Here's how the part is built. I have some questions about the finished solid (model axes, mm). A direction names the side the tool comes from. Round coordinates to 2 decimals unless told otherwise and drop trailing zeros. Write each loop counter-clockwise with the first axis right and the second up, starting at its lowest first coordinate (ties: lowest second). Pieces come first, ordered by that corner, then holes. Notation, with made-up numbers: (12.25, -34) - (36.25, -34) arc R23 cw to (36.25, -16) - close; hole circle Ø4 at (69.25, -3). An arc over 180 degrees is marked (long way). Return JSON: item names as keys, results as strings. Group by question number.
```python
from build123d import *

# Parameters (mm, degrees)
PAD_DEPTH       = 14
POCKET_DEPTH    = 13
SKETCH002_R     = 0.75
POCKET001_DEPTH = 5
SKETCH003_W     = 9
SKETCH003_H     = 54
PAD001_DEPTH    = 6
SKETCH004_R     = 1.6
POCKET002_DEPTH = 10
POCKET003_DEPTH = 4.5
CHAMFER001_SIZE = 1.5
CHAMFER003_SIZE = 0.25


with BuildPart() as part:
    # Sketch → Pad (new body)
    with BuildSketch(Plane.XY.offset(-6)):
        with BuildLine():
            ThreePointArc((-18.5, 103), (-23.449747, 100.949747), (-25.5, 96))
            Line((-25.5, 52), (-25.5, 96))
            ThreePointArc((-25.5, 52), (-23.449747, 47.050253), (-18.5, 45))
            Line((57.25, 45), (-18.5, 45))
            ThreePointArc((57.25, 45), (62.199747, 47.050253), (64.25, 52))
            Line((64.25, 96), (64.25, 52))
            ThreePointArc((64.25, 96), (62.199747, 100.949747), (57.25, 103))
            Line((-18.5, 103), (57.25, 103))
        make_face()
    extrude(amount=PAD_DEPTH)

    # Sketch001 → Pocket (cut)
    with BuildSketch(Plane.XY.offset(10)):
        with BuildLine():
            ThreePointArc((-18.5, 100.5), (-21.681981, 99.181981), (-23, 96))
            Line((-23, 52), (-23, 96))
            ThreePointArc((-23, 52), (-21.681981, 48.818019), (-18.5, 47.5))
            Line((57.25, 47.5), (-18.5, 47.5))
            ThreePointArc((57.25, 47.5), (60.431981, 48.818019), (61.75, 52))
            Line((61.75, 96), (61.75, 52))
            ThreePointArc((61.75, 96), (60.431981, 99.181981), (57.25, 100.5))
            Line((-18.5, 100.5), (57.25, 100.5))
        make_face()
    extrude(amount=-POCKET_DEPTH, mode=Mode.SUBTRACT)

    # Sketch002 → Pocket001 (cut)
    with BuildSketch(Plane(origin=(0, 104, 0), x_dir=(-1, 0, 0), z_dir=(0, 1, 0))):
        with Locations((-48.76875, 1.95)):
            Circle(SKETCH002_R)
        with Locations((-25.25, 1.95)):
            Circle(SKETCH002_R)
        with BuildLine():
            ThreePointArc((-40.17, 5.11), (-41.23066, 4.67066), (-41.67, 3.61))
            Line((-41.67, 3.05), (-41.67, 3.61))
            ThreePointArc((-41.67, 3.05), (-41.23066, 1.98934), (-40.17, 1.55))
            Line((-33.83, 1.55), (-40.17, 1.55))
            ThreePointArc((-33.83, 1.55), (-32.76934, 1.98934), (-32.33, 3.05))
            Line((-32.33, 3.61), (-32.33, 3.05))
            ThreePointArc((-32.33, 3.61), (-32.76934, 4.67066), (-33.83, 5.11))
            Line((-40.17, 5.11), (-33.83, 5.11))
        make_face()
        with BuildLine():
            ThreePointArc((-18.65, 14.05), (-19.286396, 13.786396), (-19.55, 13.15))
            Line((-19.55, 2.65), (-19.55, 13.15))
            ThreePointArc((-19.55, 2.65), (-19.286396, 2.013604), (-18.65, 1.75))
            Line((10.15, 1.75), (-18.65, 1.75))
            ThreePointArc((10.15, 1.75), (10.786396, 2.013604), (11.05, 2.65))
            Line((11.05, 13.15), (11.05, 2.65))
            ThreePointArc((11.05, 13.15), (10.786396, 13.786396), (10.15, 14.05))
            Line((-18.65, 14.05), (10.15, 14.05))
        make_face()
    extrude(amount=-POCKET001_DEPTH, mode=Mode.SUBTRACT)

    # Sketch003 → Pad001 (join)
    with BuildSketch(Plane.XY.offset(-6)):
        with Locations((-18.5, 74)):
            Rectangle(SKETCH003_W, SKETCH003_H)
        with Locations((57.25, 74)):
            Rectangle(SKETCH003_W, SKETCH003_H)
    extrude(amount=PAD001_DEPTH)

    # Sketch004 → Pocket002 (cut)
    with BuildSketch(Plane.XY):
        with Locations((-18.5, 96)):
            Circle(SKETCH004_R)
        with Locations((-18.5, 53)):
            Circle(SKETCH004_R)
        with Locations((57.25, 53)):
            Circle(SKETCH004_R)
        with Locations((57.25, 96)):
            Circle(SKETCH004_R)
    extrude(amount=-POCKET002_DEPTH, mode=Mode.SUBTRACT)

    # Sketch005 → Pocket003 (cut)
    with BuildSketch(Plane(origin=(0, 0, -6), x_dir=(-1, 0, 0), z_dir=(0, 0, -1))):
        Polygon((21.25, 94.412287), (21.25, 97.587713), (18.5, 99.175426), (15.75, 97.587713), (15.75, 94.412287), (18.5, 92.824574), align=None)
        Polygon((21.25, 51.412287), (21.25, 54.587713), (18.5, 56.175426), (15.75, 54.587713), (15.75, 51.412287), (18.5, 49.824574), align=None)
        Polygon((-54.5, 54.587713), (-57.25, 56.175426), (-60, 54.587713), (-60, 51.412287), (-57.25, 49.824574), (-54.5, 51.412287), align=None)
        Polygon((-54.5, 94.412287), (-54.5, 97.587713), (-57.25, 99.175426), (-60, 97.587713), (-60, 94.412287), (-57.25, 92.824574), align=None)
    extrude(amount=-POCKET003_DEPTH, mode=Mode.SUBTRACT)

    # Chamfer001
    chamfer001_edges = [part.edges().sort_by_distance(p)[0] for p in [
        (64.25, 74, -6),
    ]]
    chamfer(chamfer001_edges, length=CHAMFER001_SIZE)

    # Chamfer003
    chamfer003_edges = [part.edges().sort_by_distance(p)[0] for p in [
        (49.51875, 103, 1.95),
        (37, 103, 5.11),
        (26, 103, 1.95),
        (19.55, 103, 5.325),
    ]]
    chamfer(chamfer003_edges, length=CHAMFER003_SIZE)


solid = part.part
```
1) If we mould it in two halves opening along Y, with no side actions, what happens to faces 1 (the flat face through (58.61, 55.39, -3.78)), 2 (the cylindrical face through (62.15, 47, 1.66)), 3 (the flat face through (58.644, 50.63, -3.782)), 4 (the flat face through (19, 103, 0))? For each: released by +Y, released by -Y, zero draft, split by the parting line, or undercut.
2) Will these pins go through, and if not, where does the flat tip stop? pin 1 Ø2.5 at (x, y) = (-19.5, 65.5) entering from +Z; pin 2 Ø3.5 at (x, y) = (57.25, 96) entering from -Z.
3) Imagine slicing it at C-C (y = 87). Please give me the cut outline in (x, z), plus the area to 3 significant figures.
4) Imagine slicing it at A-A (y = 53). Give the number of separate pieces and of enclosed holes in the cut face, plus the area to 3 significant figures.
5) For faces 5 (the flat face through (-14, 74, -2)), 6 (the flat face through (-17.14, 55.39, -3.78)), 7 (the flat face through (64.25, 74, 2)), 8 (the conical face through (41.33, 102.873, 4.745)), which set-ups out of +Z, -Z, +X, -X, +Y, -Y let a thin tool reach every point of the face, with its end or its side?
6) I need wall thicknesses on line 1 along X through (y, z) = (96, -1); line 2 along Y through (x, z) = (57.25, -0.85); line 3 along X through (y, z) = (52.5, 3.5). Which ranges of each line are inside material? Lowest first, please.
7) Imagine slicing it at B-B (x = 8.5). Please give me the cut outline in (y, z), plus the area to 3 significant figures.
Results found:
{
 "1": {"face 1": "undercut", "face 2": "released by -Y", "face 3": "undercut", "face 4": "released by +Y"},
 "2": {"pin 1": "stops at z = 0", "pin 2": "stops at z = -1.5"},
 "3": {"outline": "(-25.5, -4.5) - (-24, -6) - (62.75, -6) - (64.25, -4.5) - (64.25, 8) - (61.75, 8) - (61.75, 0) - (52.75, 0) - (52.75, -3) - (-14, -3) - (-14, 0) - (-23, 0) - (-23, 8) - (-25.5, 8) - close", "area": "376 mm²"},
 "4": {"separate pieces": "3", "enclosed holes": "0", "area": "317 mm²"},
 "5": {"face 5": "+Z", "face 6": "-Z", "face 7": "+Z, -Z, +X, +Y, -Y", "face 8": "+Y"},
 "6": {"line 1": "x = -25.5 to -20.1, -16.9 to -14, 52.75 to 55.65, 58.85 to 64.25", "line 2": "y = 45 to 51.4, 54.6 to 94.4, 97.6 to 103", "line 3": "x = -25.5 to -23, 61.75 to 64.25"},
 "7": {"outline": "(45, -4.5) - (46.5, -6) - (101.5, -6) - (103, -4.5) - (103, 1.5) - (102.75, 1.75) - (100.5, 1.75) - (100.5, -3) - (47.5, -3) - (47.5, 8) - (45, 8) - close", "area": "211 mm²"}
}
